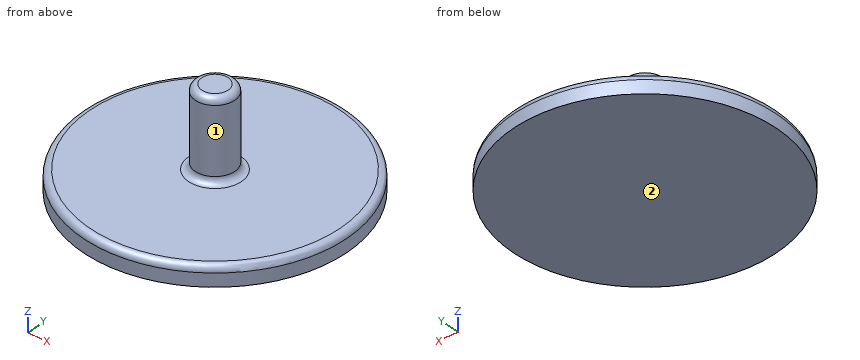
```python
from build123d import *

# Parameters (mm, degrees)
F0_R     = 20
F1_DEPTH = 3
F2_R     = 3
F3_DEPTH = 12
F4_R     = 1


with BuildPart() as f1:
    # F0 (on Top) → F1 (new body)
    with BuildSketch(Plane.XY):
        Circle(F0_R)
    extrude(amount=-F1_DEPTH)

    # F2 (on face) → F3 (join)
    with BuildSketch(Plane.XY):
        Circle(F2_R)
    extrude(amount=F3_DEPTH)

    # F4
    f4_edges = [f1.edges().sort_by_distance(p)[0] for p in [
        (-20, 0, 0),
        (-3, 0, 12),
        (-3, 0, 0),
    ]]
    fillet(f4_edges, radius=F4_R)


solid = f1.part
```
Check sheet for the modelled part. Datum: model origin and axes. Units: mm. Face numbers are marked on the shaded views. A direction names the side the tool comes from. Round coordinates to 2 decimals unless told otherwise and drop trailing zeros. Loops run counter-clockwise (first coordinate to the right, second up) from the corner with the lowest first, then second, coordinate; pieces in that order, holes last. Notation, with made-up numbers: M 38.25,54 L 64.25,54 A24 ccw 64.25,88 Z; hole C 43,85 d11. An arc over 180 degrees is marked long. Answer as a JSON object with one key per item and string values.
1. Section check C-C (z = 7.5). Record the boundary of the cut face in (x, y), plus the area to 3 significant figures.
Reply:
{"outline": "C 0,0 d6", "area": "28.3 mm²"}
2. Section check A-A (y = 0). Record the boundary of the cut face in (x, z), plus the area to 3 significant figures.
Reply:
{"outline": "M -20,-3 L 20,-3 L 20,-1 A1 ccw 19,0 L 4,0 A1 cw 3,1 L 3,11 A1 ccw 2,12 L -2,12 A1 ccw -3,11 L -3,1 A1 cw -4,0 L -19,0 A1 ccw -20,-1 Z", "area": "192 mm²"}
3. Gauge pin test, flat ends, axial feed: P1, Ø3, axis at x = -13.5, z = -0.5, coming from the +Y side; P2, Ø3, axis at x = 10, y = 13, coming from the +Z side; P3, Ø1.5, axis at y = -6, z = 0.5, coming from the +X side. Record the tip position at first contact, or that the pin passes through.
Reply:
{"P1": "stops at y = 15.95", "P2": "stops at z = 0", "P3": "stops at x = 18.75"}
4. Access from +Z, -Z, +X, -X, +Y, -Y to the whole of each face (thin tool, end or side, straight path). Record for the marked faces 1 and 2.
Reply:
{"face 1": "+Z", "face 2": "-Z, +X, -X, +Y, -Y"}
5. Scan lines: line 1 (Z direction, x = -7, y = -3); line 2 (Z direction, x = 3.5, y = 0.5); line 3 (Y direction, x = -2, z = 4). Record each from-to range of solid material in increasing order.
Reply:
{"line 1": "z = -3 to 0", "line 2": "z = -3 to 0.11", "line 3": "y = -2.24 to 2.24"}
